from build123d import *

# Parameters (mm, degrees)
CROQUIS1_W              = 175
CROQUIS1_H              = 120
SALIENTE_EXTRUIR1_DEPTH = 16
SALIENTE_EXTRUIR3_DEPTH = 41
CROQUIS7_W              = 35
CROQUIS7_H              = 16
CORTAR_EXTRUIR1_DEPTH   = 227.356466663
CROQUIS11_W             = 25
CROQUIS11_H             = 30
CORTAR_EXTRUIR2_DEPTH   = 199.447096225
CROQUIS12_R             = 25
SALIENTE_EXTRUIR4_DEPTH = 25
CROQUIS14_R             = 27.5
SALIENTE_EXTRUIR7_DEPTH = 16
SALIENTE_EXTRUIR8_START = 30
SALIENTE_EXTRUIR8_DEPTH = 30
SALIENTE_EXTRUIR9_DEPTH = 30
CROQUIS17_R             = 15
CORTAR_EXTRUIR3_DEPTH   = 210.277925257


with BuildPart() as part:
    # Croquis1 → Saliente-Extruir1 (new body)
    with BuildSketch(Plane(origin=(0, 0, 0), x_dir=(1, 0, 0), z_dir=(0, 1, 0))):
        Rectangle(CROQUIS1_W, CROQUIS1_H)
    extrude(amount=SALIENTE_EXTRUIR1_DEPTH)

    # Croquis6 → Saliente-Extruir3 (add)
    with BuildSketch(Plane.XZ):
        Polygon((87.5, 60), (162.5, 60), (187.5, 30), (187.5, -30), (162.5, -60), (87.5, -60), align=None)
    extrude(amount=-SALIENTE_EXTRUIR3_DEPTH)

    # Croquis7 → Cortar-Extruir1 (cut, through all)
    with BuildSketch(Plane.XY.offset(60)):
        with Locations((130, 8)):
            Rectangle(CROQUIS7_W, CROQUIS7_H)
    extrude(amount=-CORTAR_EXTRUIR1_DEPTH, mode=Mode.SUBTRACT)

    # Croquis11 → Cortar-Extruir2 (cut, through all)
    with BuildSketch(Plane(origin=(0, 16, 0), x_dir=(1, 0, 0), z_dir=(0, 1, 0))):
        with Locations((65.5, 0)):
            Rectangle(CROQUIS11_W, CROQUIS11_H)
    extrude(amount=-CORTAR_EXTRUIR2_DEPTH, mode=Mode.SUBTRACT)

    # Croquis12 → Saliente-Extruir4 (add)
    with BuildSketch(Plane(origin=(0, 16, 0), x_dir=(1, 0, 0), z_dir=(0, 1, 0))):
        with Locations(Location((-87.5, 0, 0), (0, 0, 270))):
            Circle(CROQUIS12_R)
    extrude(amount=SALIENTE_EXTRUIR4_DEPTH)

    # Croquis14 → Saliente-Extruir7 (add)
    with BuildSketch(Plane.XZ):
        with Locations((-87.5, 0)):
            Circle(CROQUIS14_R)
    extrude(amount=-SALIENTE_EXTRUIR7_DEPTH)

    # Croquis15 → Saliente-Extruir8 (add)
    with BuildSketch(Plane(origin=(0, 0, 0), x_dir=(-1, 0, 0), z_dir=(0, -1, 0)).offset(SALIENTE_EXTRUIR8_START)):
        with BuildLine():
            Line((87.5, 25), (87.5, -25))
            ThreePointArc((87.5, -25), (112.5, 0), (87.5, 25))
        make_face()
    extrude(amount=-SALIENTE_EXTRUIR8_DEPTH)

    # Croquis16 → Saliente-Extruir9 (add)
    with BuildSketch(Plane.XZ):
        with BuildLine():
            Line((-87.5, 30), (-87.5, -30))
            ThreePointArc((-87.5, -30), (-57.5, 0), (-87.5, 30))
        make_face()
    extrude(amount=SALIENTE_EXTRUIR9_DEPTH)

    # Croquis17 → Cortar-Extruir3 (cut, through all)
    with BuildSketch(Plane(origin=(0, 41, 0), x_dir=(1, 0, 0), z_dir=(0, 1, 0))):
        with Locations(Location((-87.5, 0, 0), (0, 0, 270))):
            Circle(CROQUIS17_R)
    extrude(amount=-CORTAR_EXTRUIR3_DEPTH, mode=Mode.SUBTRACT)


solid = part.part
Check sheet for the modelled part. Datum: model origin and axes. Units: mm. A direction names the side the tool comes from. Give positions to 0.01 mm unless a question says otherwise; leave off trailing zeros. Write each loop counter-clockwise with the first axis right and the second up, starting at its lowest first coordinate (ties: lowest second). Pieces come first, ordered by that corner, then holes. Notation, with made-up numbers: M -9.75,43 L 17.25,43 A21 cw 17.25,60 Z; hole C 34,51.5 d8. An arc over 180 degrees is marked long. Use one line per item in the form item = value.
(1) Tool access check on faces 5 (the flat face through (-87.5, 4, 43)), 6 (the cylindrical face through (-57.507, -14.79, -0.66)), 7 (the flat face through (-87.5, 4, -42)), 8 (the flat face through (87.5, 28, -1)), 9 (the flat face through (147.5, 8, 1)). Record the directions out of +Z, -Z, +X, -X, +Y, -Y that give a thin tool (end or side, any length) a straight path to the whole face; none if there is none.
Answer block:
face_5 = +Z, -X, -Y
face_6 = +X, -Y
face_7 = -Z, -X, -Y
face_8 = +Z, -Z, +Y
face_9 = +Z, -Z, -Y
(2) Section check A-A on y = 3. Record the boundary of the cut face in (x, z).
Answer block:
outline = M -87.5,-60 L 112.5,-60 L 112.5,60 L -87.5,60 L -87.5,27.5 A27.5 ccw -87.5,-27.5 Z; M 147.5,-60 L 162.5,-60 L 187.5,-30 L 187.5,30 L 162.5,60 L 147.5,60 Z; hole C -87.5,0 d30; hole M 53,-15 L 78,-15 L 78,15 L 53,15 Z
(3) Depth check by flat-ended pin: P1, Ø8, axis at y = 22.5, z = 11, coming from the -X side; P2, Ø3, axis at x = 83.5, z = 9.5, coming from the +Y side; P3, Ø7.5, axis at y = 31, z = 14.5, coming from the -X side; P4, Ø8, axis at x = -28.5, y = 17, coming from the +Z side. Enter the tip coordinate at first touch or a pass-through.
Answer block:
P1 = -111.5
P2 = 16
P3 = -110.07
P4 = 60
(4) Material ranges on line 1 along X through (y, z) = (25, 0); line 2 along X through (y, z) = (11.5, 0); line 3 along X through (y, z) = (-6.5, 0), recorded low to high.
Answer block:
line_1 = -112.5 to -102.5, -72.5 to -62.5, 87.5 to 187.5
line_2 = -115 to -102.5, -72.5 to 53, 78 to 112.5, 147.5 to 187.5
line_3 = -112.5 to -102.5, -72.5 to -57.5
(5) Section check B-B on y = 21.5. Record the boundary of the cut face in (x, z), plus the area to 3 significant figures.
Answer block:
outline = C -87.5,0 d50; M 87.5,-60 L 162.5,-60 L 187.5,-30 L 187.5,30 L 162.5,60 L 87.5,60 Z; hole C -87.5,0 d30
area = 12,500 mm2
(6) Section check C-C on z = 0. Record the boundary of the cut face in (x, y).
Answer block:
outline = M -115,0 L -112.5,0 L -112.5,-30 L -102.5,-30 L -102.5,41 L -112.5,41 L -112.5,16 L -115,16 Z; M -72.5,-30 L -57.5,-30 L -57.5,0 L 53,0 L 53,16 L -62.5,16 L -62.5,41 L -72.5,41 Z; M 78,0 L 112.5,0 L 112.5,16 L 147.5,16 L 147.5,0 L 187.5,0 L 187.5,41 L 87.5,41 L 87.5,16 L 78,16 Z
(7) Draft check along Z on faces 1 (the flat face through (65, 8, -15)), 2 (the cylindrical face through (-112.494, -15.21, 0.55)), 3 (the flat face through (65, 8, 15)), 4 (the flat face through (-98, 41, 11)). Enter one of: pulls with the +Z half, pulls with the -Z half, needs draft (parallel to the pull), parting line crosses it, or undercut.
Answer block:
face_1 = undercut
face_2 = parting line crosses it
face_3 = undercut
face_4 = needs draft
(8) Section check D-D on z = -48. Record the boundary of the cut face in (x, y).
Answer block:
outline = M -87.5,0 L 112.5,0 L 112.5,16 L 147.5,16 L 147.5,0 L 172.5,0 L 172.5,41 L 87.5,41 L 87.5,16 L -87.5,16 Z
